Check sheet for the modelled part. Datum: model origin and axes. Units: mm. Coordinates: 2 decimals unless noted, no trailing zeros. Loops run counter-clockwise (first coordinate to the right, second up) from the corner with the lowest first, then second, coordinate; pieces in that order, holes last. Notation, with made-up numbers: M -32.75,-1 L -19.75,-1 A21 cw -19.75,24 Z; hole C 89.5,32 d9. An arc over 180 degrees is marked long. Answer in a Markdown table with one row per item. Add a question column.
```python
from build123d import *

# Parameters (mm, degrees)
SKETCH_1_W          = 223.9
SKETCH_1_H          = 400
EXTRUDE_1_DEPTH     = 4.5
SKETCH_2_R          = 2
SKETCH_2_W          = 8.5
SKETCH_2_H          = 41
CUT_EXTRUDE_1_DEPTH = 10
CUT_EXTRUDE_2_REACH = 460.423
SKETCH_3_R          = 2.6
SKETCH_3_R_2        = 1.6


with BuildPart() as part:
    # 草图1 → 凸台-拉伸1 (new body)
    with BuildSketch(Plane(origin=(0, 0, 0), x_dir=(0, 0, -1), z_dir=(1, 0, 0))):
        with Locations((-111.95, 200)):
            Rectangle(SKETCH_1_W, SKETCH_1_H)
    extrude(amount=EXTRUDE_1_DEPTH)

    # 草图2 → 切除-拉伸1 (cut)
    with BuildSketch(Plane(origin=(4.5, 0, 0), x_dir=(0, 0, -1), z_dir=(1, 0, 0))):
        with Locations((-204.4, 310)):
            Circle(SKETCH_2_R)
        with Locations((-204.4, 286)):
            Circle(SKETCH_2_R)
        with Locations((-204.4, 54)):
            Circle(SKETCH_2_R)
        with Locations((-204.4, 30)):
            Circle(SKETCH_2_R)
        with Locations((-54, 384)):
            Circle(SKETCH_2_R)
        with Locations((-30, 384)):
            Circle(SKETCH_2_R)
        with Locations((-23, 320)):
            Circle(SKETCH_2_R)
        with Locations((-23, 300)):
            Circle(SKETCH_2_R)
        with Locations((-23, 50)):
            Circle(SKETCH_2_R)
        with Locations((-23, 30)):
            Circle(SKETCH_2_R)
        with Locations((-4.25, 310)):
            Rectangle(SKETCH_2_W, SKETCH_2_H)
        with Locations((-4.25, 40)):
            Rectangle(SKETCH_2_W, SKETCH_2_H)
    extrude(amount=-CUT_EXTRUDE_1_DEPTH, mode=Mode.SUBTRACT)

    # 草图3 → 切除-拉伸2 (cut, up to next)
    with BuildSketch(Plane(origin=(4.5, 0, 0), x_dir=(0, 0, -1), z_dir=(1, 0, 0)), mode=Mode.PRIVATE) as cut_extrude_2_sk1:
        with Locations((-43.9, 22)):
            Circle(SKETCH_3_R)
    cut_extrude_2_tool1 = extrude(cut_extrude_2_sk1.sketch, amount=-CUT_EXTRUDE_2_REACH, mode=Mode.PRIVATE) & part.part
    # 草图3 → 切除-拉伸2 (cut, up to next)
    with BuildSketch(Plane(origin=(4.5, 0, 0), x_dir=(0, 0, -1), z_dir=(1, 0, 0)), mode=Mode.PRIVATE) as cut_extrude_2_sk2:
        with Locations((-186.9, 22)):
            Circle(SKETCH_3_R)
    cut_extrude_2_tool2 = extrude(cut_extrude_2_sk2.sketch, amount=-CUT_EXTRUDE_2_REACH, mode=Mode.PRIVATE) & part.part
    # 草图3 → 切除-拉伸2 (cut, up to next)
    with BuildSketch(Plane(origin=(4.5, 0, 0), x_dir=(0, 0, -1), z_dir=(1, 0, 0)), mode=Mode.PRIVATE) as cut_extrude_2_sk3:
        with Locations((-43.9, 187.5)):
            Circle(SKETCH_3_R)
    cut_extrude_2_tool3 = extrude(cut_extrude_2_sk3.sketch, amount=-CUT_EXTRUDE_2_REACH, mode=Mode.PRIVATE) & part.part
    # 草图3 → 切除-拉伸2 (cut, up to next)
    with BuildSketch(Plane(origin=(4.5, 0, 0), x_dir=(0, 0, -1), z_dir=(1, 0, 0)), mode=Mode.PRIVATE) as cut_extrude_2_sk4:
        with Locations((-186.9, 187.5)):
            Circle(SKETCH_3_R)
    cut_extrude_2_tool4 = extrude(cut_extrude_2_sk4.sketch, amount=-CUT_EXTRUDE_2_REACH, mode=Mode.PRIVATE) & part.part
    # 草图3 → 切除-拉伸2 (cut, up to next)
    with BuildSketch(Plane(origin=(4.5, 0, 0), x_dir=(0, 0, -1), z_dir=(1, 0, 0)), mode=Mode.PRIVATE) as cut_extrude_2_sk5:
        with Locations((-186.9, 353)):
            Circle(SKETCH_3_R)
    cut_extrude_2_tool5 = extrude(cut_extrude_2_sk5.sketch, amount=-CUT_EXTRUDE_2_REACH, mode=Mode.PRIVATE) & part.part
    # 草图3 → 切除-拉伸2 (cut, up to next)
    with BuildSketch(Plane(origin=(4.5, 0, 0), x_dir=(0, 0, -1), z_dir=(1, 0, 0)), mode=Mode.PRIVATE) as cut_extrude_2_sk6:
        with Locations((-43.9, 353)):
            Circle(SKETCH_3_R)
    cut_extrude_2_tool6 = extrude(cut_extrude_2_sk6.sketch, amount=-CUT_EXTRUDE_2_REACH, mode=Mode.PRIVATE) & part.part
    # 草图3 → 切除-拉伸2 (cut, up to next)
    with BuildSketch(Plane(origin=(4.5, 0, 0), x_dir=(0, 0, -1), z_dir=(1, 0, 0)), mode=Mode.PRIVATE) as cut_extrude_2_sk7:
        with Locations((-115.4, 187.5)):
            Circle(SKETCH_3_R_2)
    cut_extrude_2_tool7 = extrude(cut_extrude_2_sk7.sketch, amount=-CUT_EXTRUDE_2_REACH, mode=Mode.PRIVATE) & part.part
    # 草图3 → 切除-拉伸2 (cut, up to next)
    with BuildSketch(Plane(origin=(4.5, 0, 0), x_dir=(0, 0, -1), z_dir=(1, 0, 0)), mode=Mode.PRIVATE) as cut_extrude_2_sk8:
        with Locations((-115.4, 242.5)):
            Circle(SKETCH_3_R)
    cut_extrude_2_tool8 = extrude(cut_extrude_2_sk8.sketch, amount=-CUT_EXTRUDE_2_REACH, mode=Mode.PRIVATE) & part.part
    # 草图3 → 切除-拉伸2 (cut, up to next)
    with BuildSketch(Plane(origin=(4.5, 0, 0), x_dir=(0, 0, -1), z_dir=(1, 0, 0)), mode=Mode.PRIVATE) as cut_extrude_2_sk9:
        with Locations((-115.4, 132.5)):
            Circle(SKETCH_3_R)
    cut_extrude_2_tool9 = extrude(cut_extrude_2_sk9.sketch, amount=-CUT_EXTRUDE_2_REACH, mode=Mode.PRIVATE) & part.part
    # 草图3 → 切除-拉伸2 (cut, up to next)
    with BuildSketch(Plane(origin=(4.5, 0, 0), x_dir=(0, 0, -1), z_dir=(1, 0, 0)), mode=Mode.PRIVATE) as cut_extrude_2_sk10:
        with BuildLine():
            Line((-173.9, 130), (-128.9, 130))
            ThreePointArc((-128.9, 130), (-121.828932188, 127.071067812), (-118.9, 120))
            Line((-118.9, 120), (-118.9, 90))
            ThreePointArc((-118.9, 90), (-121.828932188, 82.928932188), (-128.9, 80))
            Line((-128.9, 80), (-173.9, 80))
            ThreePointArc((-173.9, 80), (-180.971067812, 82.928932188), (-183.9, 90))
            Line((-183.9, 90), (-183.9, 120))
            ThreePointArc((-183.9, 120), (-180.971067812, 127.071067812), (-173.9, 130))
        make_face()
    cut_extrude_2_tool10 = extrude(cut_extrude_2_sk10.sketch, amount=-CUT_EXTRUDE_2_REACH, mode=Mode.PRIVATE) & part.part
    # 草图3 → 切除-拉伸2 (cut, up to next)
    with BuildSketch(Plane(origin=(4.5, 0, 0), x_dir=(0, 0, -1), z_dir=(1, 0, 0)), mode=Mode.PRIVATE) as cut_extrude_2_sk11:
        with BuildLine():
            Line((-101.9, 130), (-56.9, 130))
            ThreePointArc((-56.9, 130), (-49.828932188, 127.071067812), (-46.9, 120))
            Line((-46.9, 120), (-46.9, 90))
            ThreePointArc((-46.9, 90), (-49.828932188, 82.928932188), (-56.9, 80))
            Line((-56.9, 80), (-101.9, 80))
            ThreePointArc((-101.9, 80), (-108.971067812, 82.928932188), (-111.9, 90))
            Line((-111.9, 90), (-111.9, 120))
            ThreePointArc((-111.9, 120), (-108.971067812, 127.071067812), (-101.9, 130))
        make_face()
    cut_extrude_2_tool11 = extrude(cut_extrude_2_sk11.sketch, amount=-CUT_EXTRUDE_2_REACH, mode=Mode.PRIVATE) & part.part
    # 草图3 → 切除-拉伸2 (cut, up to next)
    with BuildSketch(Plane(origin=(4.5, 0, 0), x_dir=(0, 0, -1), z_dir=(1, 0, 0)), mode=Mode.PRIVATE) as cut_extrude_2_sk12:
        with BuildLine():
            Line((-101.9, 240), (-56.9, 240))
            ThreePointArc((-56.9, 240), (-49.828932188, 237.071067812), (-46.9, 230))
            Line((-46.9, 230), (-46.9, 200))
            ThreePointArc((-46.9, 200), (-49.828932188, 192.928932188), (-56.9, 190))
            Line((-56.9, 190), (-101.9, 190))
            ThreePointArc((-101.9, 190), (-108.971067812, 192.928932188), (-111.9, 200))
            Line((-111.9, 200), (-111.9, 230))
            ThreePointArc((-111.9, 230), (-108.971067812, 237.071067812), (-101.9, 240))
        make_face()
    cut_extrude_2_tool12 = extrude(cut_extrude_2_sk12.sketch, amount=-CUT_EXTRUDE_2_REACH, mode=Mode.PRIVATE) & part.part
    # 草图3 → 切除-拉伸2 (cut, up to next)
    with BuildSketch(Plane(origin=(4.5, 0, 0), x_dir=(0, 0, -1), z_dir=(1, 0, 0)), mode=Mode.PRIVATE) as cut_extrude_2_sk13:
        with BuildLine():
            Line((-101.9, 350), (-56.9, 350))
            ThreePointArc((-56.9, 350), (-49.828932188, 347.071067812), (-46.9, 340))
            Line((-46.9, 340), (-46.9, 310))
            ThreePointArc((-46.9, 310), (-49.828932188, 302.928932188), (-56.9, 300))
            Line((-56.9, 300), (-101.9, 300))
            ThreePointArc((-101.9, 300), (-108.971067812, 302.928932188), (-111.9, 310))
            Line((-111.9, 310), (-111.9, 340))
            ThreePointArc((-111.9, 340), (-108.971067812, 347.071067812), (-101.9, 350))
        make_face()
    cut_extrude_2_tool13 = extrude(cut_extrude_2_sk13.sketch, amount=-CUT_EXTRUDE_2_REACH, mode=Mode.PRIVATE) & part.part
    # 草图3 → 切除-拉伸2 (cut, up to next)
    with BuildSketch(Plane(origin=(4.5, 0, 0), x_dir=(0, 0, -1), z_dir=(1, 0, 0)), mode=Mode.PRIVATE) as cut_extrude_2_sk14:
        with BuildLine():
            Line((-173.9, 240), (-128.9, 240))
            ThreePointArc((-128.9, 240), (-121.828932188, 237.071067812), (-118.9, 230))
            Line((-118.9, 230), (-118.9, 200))
            ThreePointArc((-118.9, 200), (-121.828932188, 192.928932188), (-128.9, 190))
            Line((-128.9, 190), (-173.9, 190))
            ThreePointArc((-173.9, 190), (-180.971067812, 192.928932188), (-183.9, 200))
            Line((-183.9, 200), (-183.9, 230))
            ThreePointArc((-183.9, 230), (-180.971067812, 237.071067812), (-173.9, 240))
        make_face()
    cut_extrude_2_tool14 = extrude(cut_extrude_2_sk14.sketch, amount=-CUT_EXTRUDE_2_REACH, mode=Mode.PRIVATE) & part.part
    # 草图3 → 切除-拉伸2 (cut, up to next)
    with BuildSketch(Plane(origin=(4.5, 0, 0), x_dir=(0, 0, -1), z_dir=(1, 0, 0)), mode=Mode.PRIVATE) as cut_extrude_2_sk15:
        with BuildLine():
            Line((-173.9, 350), (-128.9, 350))
            ThreePointArc((-128.9, 350), (-121.828932188, 347.071067812), (-118.9, 340))
            Line((-118.9, 340), (-118.9, 310))
            ThreePointArc((-118.9, 310), (-121.828932188, 302.928932188), (-128.9, 300))
            Line((-128.9, 300), (-173.9, 300))
            ThreePointArc((-173.9, 300), (-180.971067812, 302.928932188), (-183.9, 310))
            Line((-183.9, 310), (-183.9, 340))
            ThreePointArc((-183.9, 340), (-180.971067812, 347.071067812), (-173.9, 350))
        make_face()
    cut_extrude_2_tool15 = extrude(cut_extrude_2_sk15.sketch, amount=-CUT_EXTRUDE_2_REACH, mode=Mode.PRIVATE) & part.part
    add(cut_extrude_2_tool1.solids().sort_by_distance((4.5, 22, 43.9))[0], mode=Mode.SUBTRACT)
    add(cut_extrude_2_tool2.solids().sort_by_distance((4.5, 22, 186.9))[0], mode=Mode.SUBTRACT)
    add(cut_extrude_2_tool3.solids().sort_by_distance((4.5, 187.5, 43.9))[0], mode=Mode.SUBTRACT)
    add(cut_extrude_2_tool4.solids().sort_by_distance((4.5, 187.5, 186.9))[0], mode=Mode.SUBTRACT)
    add(cut_extrude_2_tool5.solids().sort_by_distance((4.5, 353, 186.9))[0], mode=Mode.SUBTRACT)
    add(cut_extrude_2_tool6.solids().sort_by_distance((4.5, 353, 43.9))[0], mode=Mode.SUBTRACT)
    add(cut_extrude_2_tool7.solids().sort_by_distance((4.5, 187.5, 115.4))[0], mode=Mode.SUBTRACT)
    add(cut_extrude_2_tool8.solids().sort_by_distance((4.5, 242.5, 115.4))[0], mode=Mode.SUBTRACT)
    add(cut_extrude_2_tool9.solids().sort_by_distance((4.5, 132.5, 115.4))[0], mode=Mode.SUBTRACT)
    add(cut_extrude_2_tool10.solids().sort_by_distance((4.5, 105, 151.4))[0], mode=Mode.SUBTRACT)
    add(cut_extrude_2_tool11.solids().sort_by_distance((4.5, 105, 79.4))[0], mode=Mode.SUBTRACT)
    add(cut_extrude_2_tool12.solids().sort_by_distance((4.5, 215, 79.4))[0], mode=Mode.SUBTRACT)
    add(cut_extrude_2_tool13.solids().sort_by_distance((4.5, 325, 79.4))[0], mode=Mode.SUBTRACT)
    add(cut_extrude_2_tool14.solids().sort_by_distance((4.5, 215, 151.4))[0], mode=Mode.SUBTRACT)
    add(cut_extrude_2_tool15.solids().sort_by_distance((4.5, 325, 151.4))[0], mode=Mode.SUBTRACT)


solid = part.part
```
Q1. Cross-section at C-C (z = 179). Record the cut outline in (x, y), plus the area to 3 significant figures.
Q2. Mould release check, pull along Y, two halves, no side actions. Record for faces 1 (the face through (2.28, 127.15, 49.91)), 2 (the face through (4.5, 203, 114)): released by +Y, released by -Y, zero draft, split by the parting line, or undercut.
Q3. Cross-section at A-A (z = 133). Record the cut outline in (x, y), plus the area to 4 significant figures.
Q4. Cross-section at B-B (x = 2.2). Count the separate pieces of the cut face and the enclosed holes in it, plus the area to 3 significant figures.
Q5. Thickness scan on L1, parallel to Y at x = 2.75, z = 23; L2, parallel to Y at x = 4.15, z = 96.5; L3, parallel to Z at x = 1.9, y = 227.5. Record the ranges inside material, lowest first.
Answer key:
| question | item | result |
|---|---|---|
| 1 | outline | M 0,0 L 4.5,0 L 4.5,81.4 L 0,81.4 Z; M 0,128.6 L 4.5,128.6 L 4.5,191.4 L 0,191.4 Z; M 0,238.6 L 4.5,238.6 L 4.5,301.4 L 0,301.4 Z; M 0,348.6 L 4.5,348.6 L 4.5,400 L 0,400 Z |
| 1 | area | 1,160 mm^2 |
| 2 | face 1 | undercut |
| 2 | face 2 | zero draft |
| 3 | outline | M 0,0 L 4.5,0 L 4.5,80 L 0,80 Z; M 0,130 L 4.5,130 L 4.5,190 L 0,190 Z; M 0,240 L 4.5,240 L 4.5,300 L 0,300 Z; M 0,350 L 4.5,350 L 4.5,400 L 0,400 Z |
| 3 | area | 1,125 mm^2 |
| 4 | separate pieces | 1 |
| 4 | enclosed holes | 25 |
| 4 | area | 69,600 mm^2 |
| 5 | L1 | 0 to 28, 32 to 48, 52 to 298, 302 to 318, 322 to 400 |
| 5 | L2 | 0 to 80, 130 to 190, 240 to 300, 350 to 400 |
| 5 | L3 | 0 to 46.9, 111.9 to 118.9, 183.9 to 223.9 |
